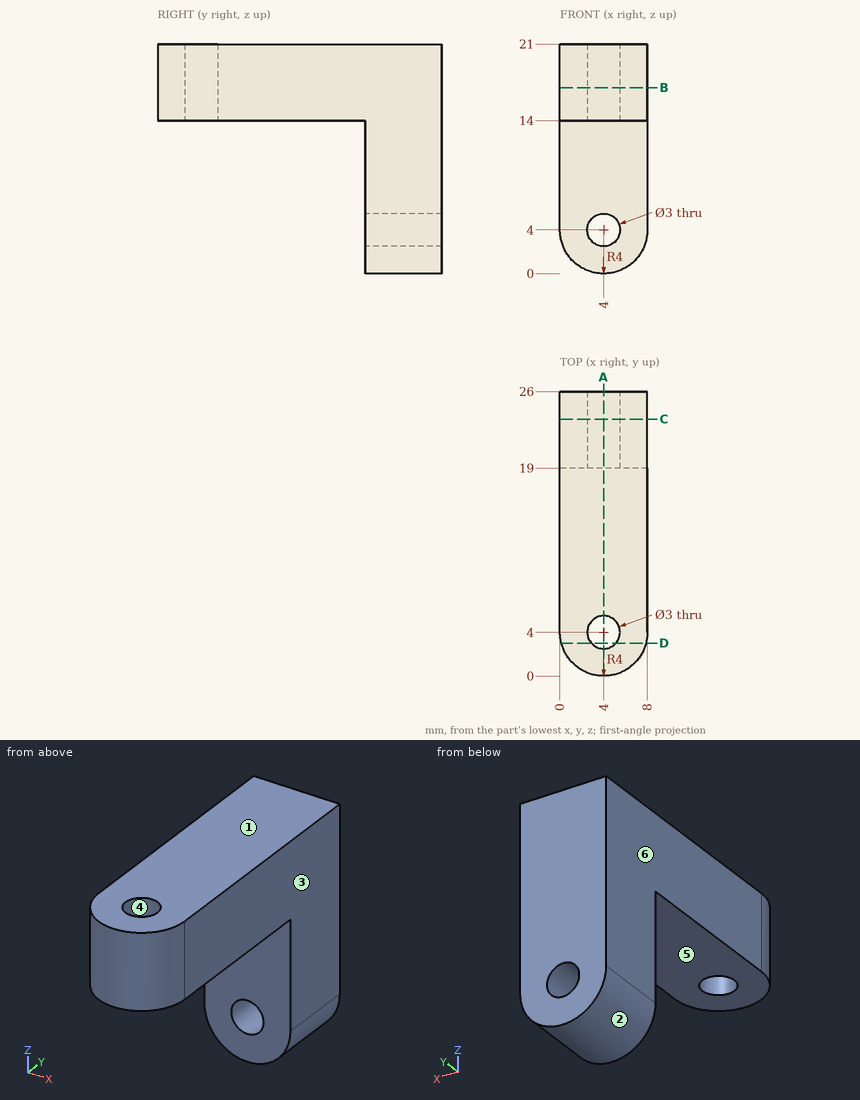
Design review of the part shown in the three views and the two pictorial views. Dimensions are in mm from the part's minimum x, y and z. A direction names the side the tool comes from. Round coordinates to 2 decimals unless told otherwise and drop trailing zeros. Write each loop counter-clockwise with the first axis right and the second up, starting at its lowest first coordinate (ties: lowest second). Pieces come first, ordered by that corner, then holes. Notation, with made-up numbers: M 42.5,-21 L 48.5,-21 A18 cw 48.5,5 Z; hole C 87.5,-4.5 d10. An arc over 180 degrees is marked long. One line per item, written item: value. Start each with the question number.
1. For the marked faces 5 and 6, list the 3-axis set-ups (+Z, -Z, +X, -X, +Y, -Y) from which the entire face can be reached by the end or side of a thin tool; tool diameter is ignored.
2. Take a section at D-D on y = 3. State the section outline as (x, z) points.
3. Take a section at B-B on z = 17. State the section outline as (x, y) points, then the cut area to 3 significant figures.
4. Clearance check with flat-ended pins moving along their axes: P1, Ø3, axis at x = 3.5, y = 13, coming from the -Z side; P2, Ø2, axis at x = 7, z = 5.5, coming from the -Y side. State where each tip first meets the part, or that it passes through.
5. Take a section at C-C on y = 23.5. State the section outline as (x, z) points, then the cut area to 3 significant figures.
6. Draft analysis for pull direction X (two halves, no side actions). For the marked faces 1, 2, 3 and 4, state which applies: pulls with the +X half, pulls with the -X half, needs draft (parallel to the pull), parting line crosses it, or undercut.
7. To check wall thickness, follow probe 1 along Y at (x, z) = (4, 19); probe 2 along X at (y, z) = (21.5, 4); probe 3 along Z at (x, y) = (4, 21). State the ranges of each line that lie inside material, in increasing order. Write a range as from..to.
8. Take a section at A-A on x = 4. State the section outline as (y, z) points, then the cut area to 3 significant figures.
Computed:
1. face 5: -Z, +X, -X, -Y
1. face 6: +Z, -Z, -X, +Y, -Y
2. outline: M 0.13,14 L 2.88,14 L 2.88,21 L 0.13,21 Z; M 5.12,14 L 7.87,14 L 7.87,21 L 5.12,21 Z
3. outline: M 0,4 A4 ccw 8,4 L 8,26 L 0,26 Z; hole C 4,4 d3
3. area: 194 mm²
4. P1: stops at z = 14
4. P2: stops at y = 19
5. outline: M 0,4 A4 ccw 8,4 L 8,21 L 0,21 Z; hole C 4,4 d3
5. area: 154 mm²
6. face 1: needs draft
6. face 2: parting line crosses it
6. face 3: pulls with the +X half
6. face 4: undercut
7. probe 1: y = 0..2.5, 5.5..26
7. probe 2: x = 0..2.5, 5.5..8
7. probe 3: z = 0..2.5, 5.5..21
8. outline: M 0,14 L 2.5,14 L 2.5,21 L 0,21 Z; M 5.5,14 L 19,14 L 19,5.5 L 26,5.5 L 26,21 L 5.5,21 Z; M 19,0 L 26,0 L 26,2.5 L 19,2.5 Z
8. area: 238 mm²
